from build123d import *

# Parameters (mm, degrees)
F0_R     = 0.69
F0_R_2   = 0.635
F1_DEPTH = 24.2
F0_R_3   = 0.5
F2_DEPTH = 25.5
F3_DEPTH = 1
F4_R     = 0.6


# Not quite as in the source:
# - a fillet or chamfer that OpenCascade refuses, or shapes differently, is made with other operations: its cross-section is extruded or revolved along the edge and cut away or added


with BuildPart() as f1:
    # F0 (on Top) → F1 (new body)
    with BuildSketch(Plane.XY):
        Circle(F0_R)
        Circle(F0_R_2, mode=Mode.SUBTRACT)
    extrude(amount=F1_DEPTH)

    # F0 (on Top) → F2 (join)
    with BuildSketch(Plane.XY):
        Circle(F0_R_2)
        Circle(F0_R_3, mode=Mode.SUBTRACT)
    extrude(amount=F2_DEPTH)

    # F0 (on Top) → F3 (join)
    with BuildSketch(Plane.XY):
        Circle(F0_R)
        Circle(F0_R_2, mode=Mode.SUBTRACT)
        Circle(F0_R_2)
        Circle(F0_R_3, mode=Mode.SUBTRACT)
        Circle(F0_R_3)
    extrude(amount=F3_DEPTH)

    # F4
    f4_edges = [f1.edges().sort_by_distance(p)[0] for p in [
        (-0.69, 0, 0),
    ]]
    fillet(f4_edges, radius=F4_R)

    # F5: fillet of radius 0.2 on 2 edges, made by hand

    # F5_s1 → F5_t2 (revolve, cut)
    with BuildSketch(Plane.XZ):
        with BuildLine():
            ThreePointArc((0.69, 24.0622502269), (0.6757417562, 24.1364122117), (0.635, 24.2))
            Line((0.635, 24.2), (0.69, 24.2))
            Line((0.69, 24.2), (0.69, 24.0622502269))
        make_face()
    revolve(axis=Axis((0, 0, 24.2), (0, 0, 1)), mode=Mode.SUBTRACT)

    # F5_s3 → F5_t4 (revolve, cut)
    with BuildSketch(Plane.XZ):
        with BuildLine():
            ThreePointArc((0.635, 25.3108571968), (0.597788206, 25.4270466972), (0.5, 25.5))
            Line((0.5, 25.5), (0.635, 25.5))
            Line((0.635, 25.5), (0.635, 25.3108571968))
        make_face()
    revolve(axis=Axis((0, 0, 25.5), (0, 0, 1)), mode=Mode.SUBTRACT)


solid = f1.part
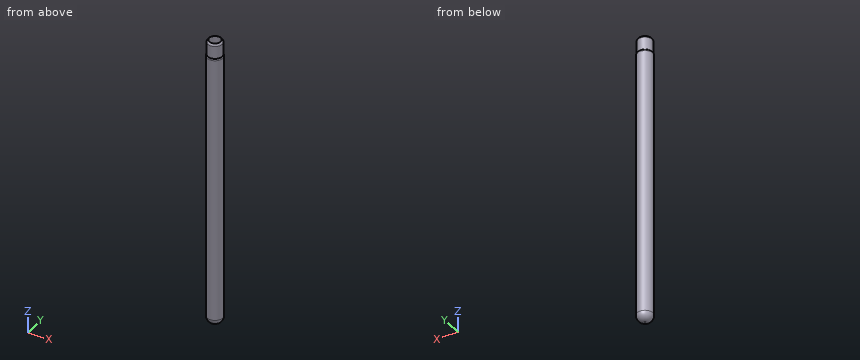
Could you check a few things on this model? Use its own coordinates, in mm. Give positions to 0.01 mm unless a question says otherwise; leave off trailing zeros. Order: outer loops, then holes, each group sorted by start corner. A loop starts at its lowest first (then second) coordinate and runs counter-clockwise, first axis right, second up.
Item 1: If we section it at A-A, the plane z = 5.5: Write out the boundary of the cut face in (x, y), plus the area to 3 significant figures.
Item 2: I'm going to push a flat-ended pin straight in: pin 1 (0.8 mm diameter, centred on x = 0, y = 0, fed in from +Z). Where does the tip first touch, or does it pass through?
Item 3: I need wall thicknesses on line 1 (Y direction, x = 0, z = 11); line 2 (X direction, y = -0.35, z = 22.25); line 3 (Z direction, x = 0.15, y = 0.05). Which ranges of each line are inside material? Lowest first, please.
Values:
1. outline: circle Ø1.38 at (0, 0); hole circle Ø1 at (0, 0)
1. area: 0.710 mm2
2. pin 1: stops at z = 1
3. line 1: y = -0.69 to -0.5, 0.5 to 0.69
3. line 2: x = -0.59 to -0.36, 0.36 to 0.59
3. line 3: z = 0 to 1
